CAD build for the part. Positions are in the model's coordinates, mm. Face numbers are marked on the shaded views. A direction names the side the tool comes from. Coordinates: 2 decimals unless noted, no trailing zeros. Loops run counter-clockwise (first coordinate to the right, second up) from the corner with the lowest first, then second, coordinate; pieces in that order, holes last. Notation, with made-up numbers: M 74,82.5 L 101,82.5 A24 cw 101,114.5 Z; hole C 3,-31.75 d5. An arc over 180 degrees is marked long. Answer as a JSON object with one key per item and string values. Group by question number.
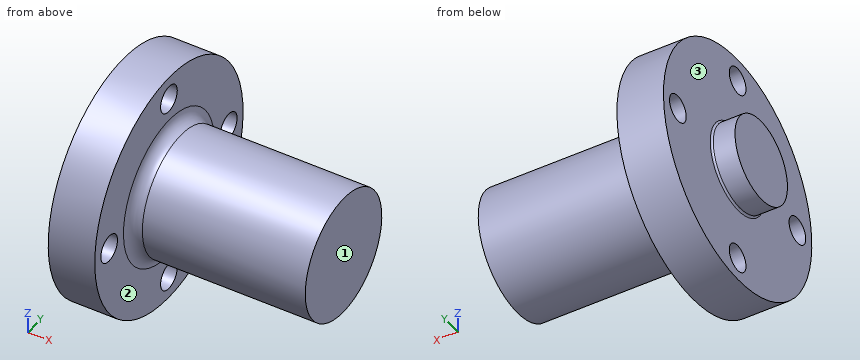
```python
from build123d import *

# Parameters (mm, degrees)
SKETCH1_R           = 24.6126
BOSS_EXTRUDE1_DEPTH = 9.525
BOSS_EXTRUDE2_START = 9.525
SKETCH2_R           = 12.7
BOSS_EXTRUDE2_DEPTH = 35.7124
SKETCH3_R           = 8.7122
BOSS_EXTRUDE4_DEPTH = 4.826
SKETCH4_R           = 2.7686
CUT_EXTRUDE2_DEPTH  = 58.078739617
FILLET1_R           = 0.381
FILLET2_R           = 2.3876


with BuildPart() as part:
    # Sketch1 → Boss-Extrude1 (new body)
    with BuildSketch(Plane.YZ):
        with Locations(Location((0, 0, 0), (0, 0, 270))):
            Circle(SKETCH1_R)
    extrude(amount=BOSS_EXTRUDE1_DEPTH)

    # Sketch2 → Boss-Extrude2 (add)
    with BuildSketch(Plane.YZ.offset(BOSS_EXTRUDE2_START)):
        with Locations(Location((0, 0, 0), (0, 0, 270))):
            Circle(SKETCH2_R)
    extrude(amount=BOSS_EXTRUDE2_DEPTH)

    # Sketch3 → Boss-Extrude4 (add)
    with BuildSketch(Plane.YZ):
        with Locations(Location((0, 0, 0), (0, 0, 270))):
            Circle(SKETCH3_R)
    extrude(amount=-BOSS_EXTRUDE4_DEPTH)

    # Sketch4 → Cut-Extrude2 (cut, through all)
    with BuildSketch(Plane.YZ):
        with Locations(Location((0, 19.8374, 0), (0, 0, 270))):
            Circle(SKETCH4_R)
        with Locations(Location((19.8374, 0, 0), (0, 0, 270))):
            Circle(SKETCH4_R)
        with Locations(Location((0, -19.8374, 0), (0, 0, 270))):
            Circle(SKETCH4_R)
        with Locations(Location((-19.8374, 0, 0), (0, 0, 270))):
            Circle(SKETCH4_R)
    extrude(amount=CUT_EXTRUDE2_DEPTH, mode=Mode.SUBTRACT)

    # Fillet1
    fillet1_edges = [part.edges().sort_by_distance(p)[0] for p in [
        (0, 0, 8.7122),
    ]]
    fillet(fillet1_edges, radius=FILLET1_R)

    # Fillet2
    fillet2_edges = [part.edges().sort_by_distance(p)[0] for p in [
        (9.525, 0, 12.7),
    ]]
    fillet(fillet2_edges, radius=FILLET2_R)


solid = part.part
```
Item 1: Slice it at A-A, the plane z = 0. Write the cut outline in (x, y) (3 decimals), then the cut area to 3 significant figures.
Item 2: Pin check, flat tips, straight feed: pin 1 (5 mm diameter, centred on y = -13, z = -4.5, fed in from -X); pin 2 (8 mm diameter, centred on x = 26, y = -8, fed in from +Z); pin 3 (3 mm diameter, centred on x = 4, z = 6, fed in from +Y); pin 4 (4.5 mm diameter, centred on y = 0, z = 19.84, fed in from +X). Stop position of each tip, or through.
Item 3: Slice it at D-D, the plane x = 30. Write the cut outline in (y, z).
Item 4: Tool access for the marked faces 1, 2 and 3: list every direction of +Z, -Z, +X, -X, +Y, -Y with a clear straight run to the whole face (end or side of a thin tool).
Item 5: Drill centre lines: L1, parallel to Y at x = 7, z = 0; L2, parallel to X at y = -20.5, z = 9.5 (3 decimals); L3, parallel to X at y = 9.5, z = -4. Where is each one in solid material? Low to high. Write a range as from..to.
Item 6: Slice it at C-C, the plane z = -20. Write the cut outline in (x, y) (3 decimals), then the cut area to 3 significant figures.
Computed:
{
 "1": {"outline": "M -4.826,-8.712 L -0.381,-8.712 A0.381 cw 0,-9.093 L 0,-17.069 L 9.525,-17.069 L 9.525,-15.088 A2.388 cw 11.913,-12.7 L 45.237,-12.7 L 45.237,12.7 L 11.913,12.7 A2.388 cw 9.525,15.088 L 9.525,17.069 L 0,17.069 L 0,9.093 A0.381 cw -0.381,8.712 L -4.826,8.712 Z; M 0,-24.613 L 9.525,-24.613 L 9.525,-22.606 L 0,-22.606 Z; M 0,22.606 L 9.525,22.606 L 9.525,24.613 L 0,24.613 Z", "area": "1,360 mm2"},
 "2": {"pin 1": "x = 0", "pin 2": "z = 12.05", "pin 3": "y = 24.2", "pin 4": "through"},
 "3": {"outline": "C 0,0 d25.4"},
 "4": {"face 1": "+Z, -Z, +X, +Y, -Y", "face 2": "+X", "face 3": "-X"},
 "5": {"L1": "-24.61..-22.61, -17.07..17.07, 22.61..24.61", "L2": "0..9.525", "L3": "0..45.24"},
 "6": {"outline": "M 0,-14.345 L 9.525,-14.345 L 9.525,-2.764 L 0,-2.764 Z; M 0,2.764 L 9.525,2.764 L 9.525,14.345 L 0,14.345 Z", "area": "221 mm2"}
}
